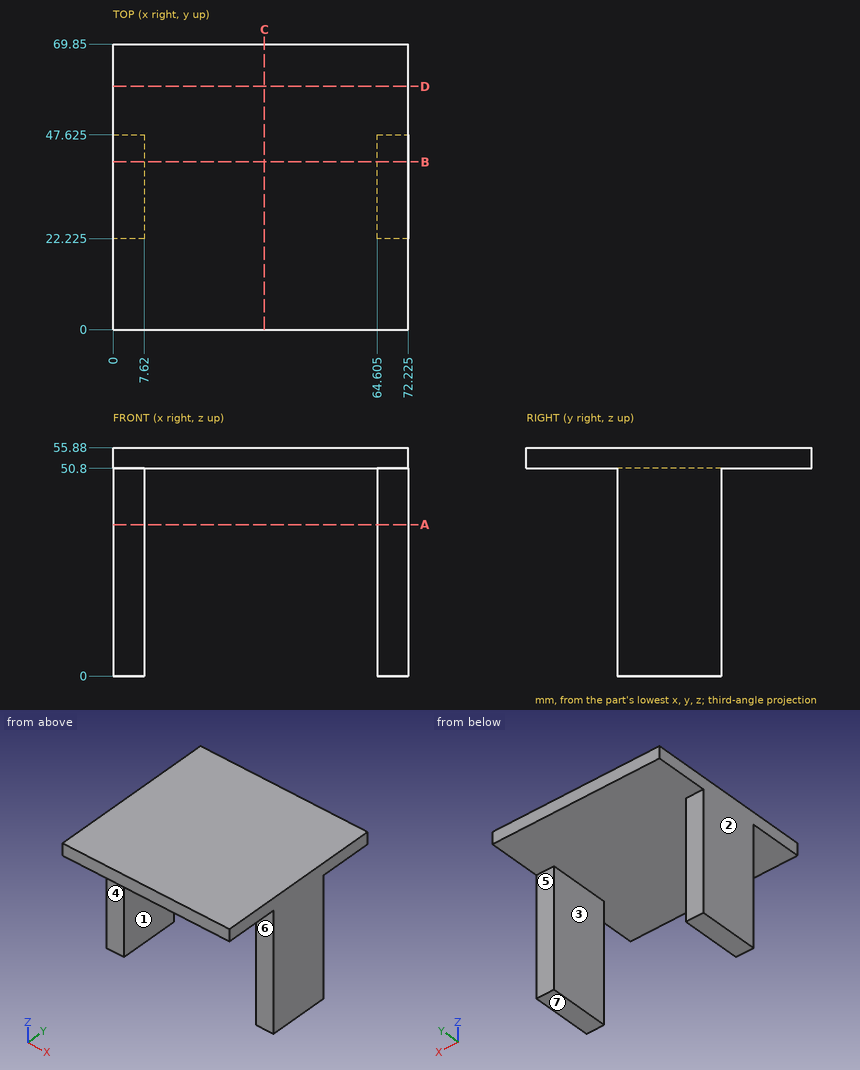
Part print with two shaded views. Sizes in mm from the minimum x, y, z corner. A direction names the side the tool comes from. Coordinates: 2 decimals unless noted, no trailing zeros. Write each loop counter-clockwise with the first axis right and the second up, starting at its lowest first coordinate (ties: lowest second). Pieces come first, ordered by that corner, then holes. Notation, with made-up numbers: (66.5, 82.5) - (76.5, 82.5) arc R26 ccw to (76.5, 96.5) - close; hole circle Ø6 at (49, 89). An arc over 180 degrees is marked (long way). Put each result on its own line as item: value.
1. Band-saw the part on B-B (y = 41). Write the cut outline in (x, z) (3 decimals).
Final values:
outline: (0, 0) - (7.62, 0) - (7.62, 50.8) - (64.605, 50.8) - (64.605, 0) - (72.225, 0) - (72.225, 55.88) - (0, 55.88) - close
2. Band-saw the part on D-D (y = 59.5). Write the cut outline in (x, z) (3 decimals).
Final values:
outline: (0, 50.8) - (72.225, 50.8) - (72.225, 55.88) - (0, 55.88) - close
3. Band-saw the part on A-A (z = 37). Write the cut outline in (x, y) (3 decimals), then the cut area to 3 significant figures.
Final values:
outline: (0, 22.225) - (7.62, 22.225) - (7.62, 47.625) - (0, 47.625) - close; (64.605, 22.225) - (72.225, 22.225) - (72.225, 47.625) - (64.605, 47.625) - close
area: 387 mm²
4. 3-axis set-ups, long thin cutter, end or side, ignore diameter. For the marked faces 5, 6 and 7: which of +Z, -Z, +X, -X, +Y, -Y reach the whole face in a straight line?
Final values:
face 5: -Z, +X, -X, +Y
face 6: -Z, +X, -X, -Y
face 7: -Z, +X, -X, +Y, -Y
5. Flat gauge pins, fed straight in: pin 1 Ø8.5 at (x, z) = (3.5, 32) entering from +Y (3 decimals); pin 2 Ø6 at (x, y) = (55, 53.5) entering from -Z; pin 3 Ø7.5 at (y, z) = (35.5, 28.5) entering from -X; pin 4 Ø8.5 at (x, z) = (67, 19) entering from -Y (3 decimals). Where does each tip first touch, or does it go through?
Final values:
pin 1: stops at y = 47.625
pin 2: stops at z = 50.8
pin 3: stops at x = 0
pin 4: stops at y = 22.225
6. Two-plate mould, pull along X, no slides. Class the marked faces 1, 2, 3 and 4: +X half, -X half, draft (parallel to the pull), parting line (faces both ways), or undercut.
Final values:
face 1: undercut
face 2: -X half
face 3: undercut
face 4: draft
7. Probe line 1 along X through (y, z) = (24.5, 33.5) (3 decimals); line 2 along Z through (x, y) = (28.5, 52); line 3 along Y through (x, z) = (66, 11.5) (3 decimals). List the from-to ranges inside material, lowest first. Write a range as [from, to].
Final values:
line 1: x = [0, 7.62], [64.605, 72.225]
line 2: z = [50.8, 55.88]
line 3: y = [22.225, 47.625]
8. Band-saw the part on C-C (x = 37). Write the cut outline in (y, z), then the cut area to 3 significant figures.
Final values:
outline: (0, 50.8) - (69.85, 50.8) - (69.85, 55.88) - (0, 55.88) - close
area: 355 mm²
